Input: part model. Units: mm. Frame: model coordinates. Face numbers are marked on the shaded views. A direction names the side the tool comes from. Coordinates: 2 decimals unless noted, no trailing zeros. Loops run counter-clockwise (first coordinate to the right, second up) from the corner with the lowest first, then second, coordinate; pieces in that order, holes last.
Item 1: Section C-C on z = 28.5. Return loops of the section in (x, y), and give its area (3 significant figures).
Item 2: Section A-A on x = -28. Return loops of the section in (y, z) (3 decimals).
Item 3: Contact query for flat-ended pins moving along their axis: P1, Ø10, axis at y = -37.5, z = 14, coming from the +X side; P2, Ø1.5, axis at x = -14.5, z = 31, coming from the +Y side; P3, Ø6, axis at y = -45, z = 67, coming from the -X side; P4, Ø4, axis at x = -11, y = -83.5, coming from the +Z side. Output: stop coordinate, or through.
Item 4: Pull-direction query (Y, two-part tool) for the marked faces 4, 5 and 6; classes: released by +Y, released by -Y, zero draft, split by the parting line, or undercut.
Item 5: Ray query, line 1 along X through (y, z) = (-38, 21); line 2 along X through (y, z) = (-38, 25); line 3 along Y through (x, z) = (-42, 6.5). Return the intervals inside material, ascending.
Item 6: Reachability of the marked faces 1, 2 and 3 from +Z, -Z, +X, -X, +Y, -Y: full face, straight path, thin tool, end or side. Return the list, or none.
Item 7: Section D-D on y = -38.1. Return loops of the section in (x, z), and give its area (3 significant figures).
Item 8: Section B-B on y = 6. Return loops of the section in (x, z).
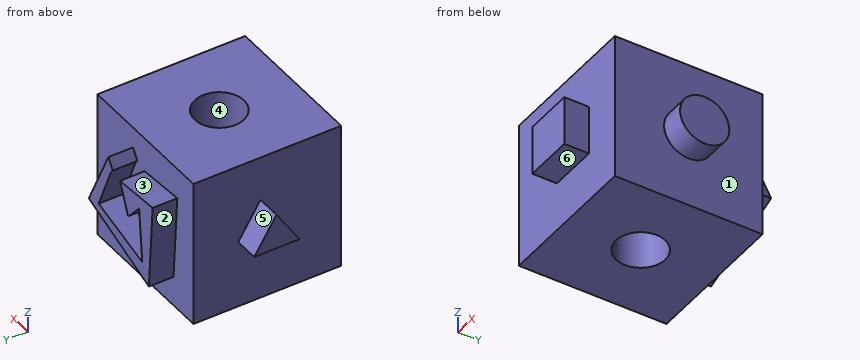
```python
from build123d import *

# Parameters (mm, degrees)
F0_W      = 76.2
F0_H      = 76.2
F1_DEPTH  = 76.2
F2_W      = 25.4
F2_H      = 25.4
F3_DEPTH  = 12.7
F4_R      = 12.7
F5_DEPTH  = 12.7
F7_D      = 25.4
F9_DEPTH  = 12.7
F11_DEPTH = 12.7


with BuildPart() as f1:
    # F0 (on Front) → F1 (new body)
    with BuildSketch(Plane.XZ):
        with Locations((-17.554368, 37.4227)):
            Rectangle(F0_W, F0_H)
    extrude(amount=F1_DEPTH)

    # F2 (on face) → F3 (join)
    with BuildSketch(Plane.XZ.offset(76.2)):
        with Locations((-12.7, 37.4227)):
            Rectangle(F2_W, F2_H)
    extrude(amount=F3_DEPTH)

    # F4 (on face) → F5 (join)
    with BuildSketch(Plane.YZ.offset(20.545632)):
        with Locations((-38.1, 37.4227)):
            Circle(F4_R)
    extrude(amount=F5_DEPTH)

    # F7 (through all)
    with Locations(Plane.XY.offset(75.5227)):
        with Locations((-17.554368, -38.1)):
            Hole(F7_D / 2)

    # F8 (on face) → F9 (join)
    with BuildSketch(Plane(origin=(-55.654368, 0, 0), x_dir=(0, -1, 0), z_dir=(-1, 0, 0))):
        Polygon((46.53557, 34.294344), (34.590948, 52.495673), (23.120321, 34.294344), align=None)
    extrude(amount=F9_DEPTH)

    # F10 (on face) → F11 (join)
    with BuildSketch(Plane(origin=(0, 0, 0), x_dir=(-1, 0, 0), z_dir=(0, 1, 0))):
        Polygon((9.674511, 57.68837), (11.108014, 59.571687), (7.686859, 64.753473), (-7.840106, 32.313734), (39.842051, 14.852335), (42.817518, 59.571687), (16.907275, 57.68837), (23.262199, 42.698413), (24.467854, 43.567646), (32.056715, 52.438211), (34.606893, 24.81661), (0, 34.446057), align=None)
    extrude(amount=F11_DEPTH)


solid = f1.part
```
Results found:
1. outline: (-55.65, -76.2) - (-25.4, -76.2) - (-25.4, -88.9) - (0, -88.9) - (0, -76.2) - (20.55, -76.2) - (20.55, -47.14) - (33.25, -47.14) - (33.25, -29.06) - (20.55, -29.06) - (20.55, 0) - (-2.57, 0) - (-2.57, 12.7) - (-21.37, 12.7) - (-21.37, 0) - (-34.27, 0) - (-34.27, 12.7) - (-40.75, 12.7) - (-40.75, 0) - (-55.65, 0) - close; hole circle Ø25.4 at (-17.55, -38.1)
1. area: 6,170 mm2
2. outline: (-76.2, -0.677) - (-45.323, -0.677) - (-45.323, 75.523) - (-76.2, 75.523) - close; (-30.877, -0.677) - (0, -0.677) - (0, 19.189) - (12.7, 19.189) - (12.7, 26.655) - (0, 26.655) - (0, 47.696) - (12.7, 47.696) - (12.7, 58.495) - (0, 58.495) - (0, 75.523) - (-30.877, 75.523) - close
3. P1: stops at x = 20.55
3. P2: stops at y = 12.7
3. P3: stops at x = -55.65
3. P4: stops at z = 50.12
4. face 4: undercut
4. face 5: released by +Y
4. face 6: zero draft
5. line 1: x = -55.65 to -30.25, -4.85 to 20.55
5. line 2: x = -55.65 to -30.25, -4.85 to 33.25
5. line 3: y = -76.2 to 0
6. face 1: +X
6. face 2: -Z, -X, +Y
6. face 3: +Z, +Y
7. outline: (-68.35, 34.29) - (-55.65, 34.29) - (-55.65, -0.68) - (-30.25, -0.68) - (-30.25, 75.52) - (-55.65, 75.52) - (-55.65, 47.15) - (-68.35, 47.15) - close; (-4.85, -0.68) - (20.55, -0.68) - (20.55, 24.72) - (33.25, 24.72) - (33.25, 50.12) - (20.55, 50.12) - (20.55, 75.52) - (-4.85, 75.52) - close
7. area: 4,360 mm2
8. outline: (-42.82, 59.57) - (-39.84, 14.85) - (7.84, 32.31) - (-7.69, 64.75) - (-11.11, 59.57) - (-9.67, 57.69) - (0, 34.45) - (-34.61, 24.82) - (-32.06, 52.44) - (-24.47, 43.57) - (-23.26, 42.7) - (-16.91, 57.69) - close
